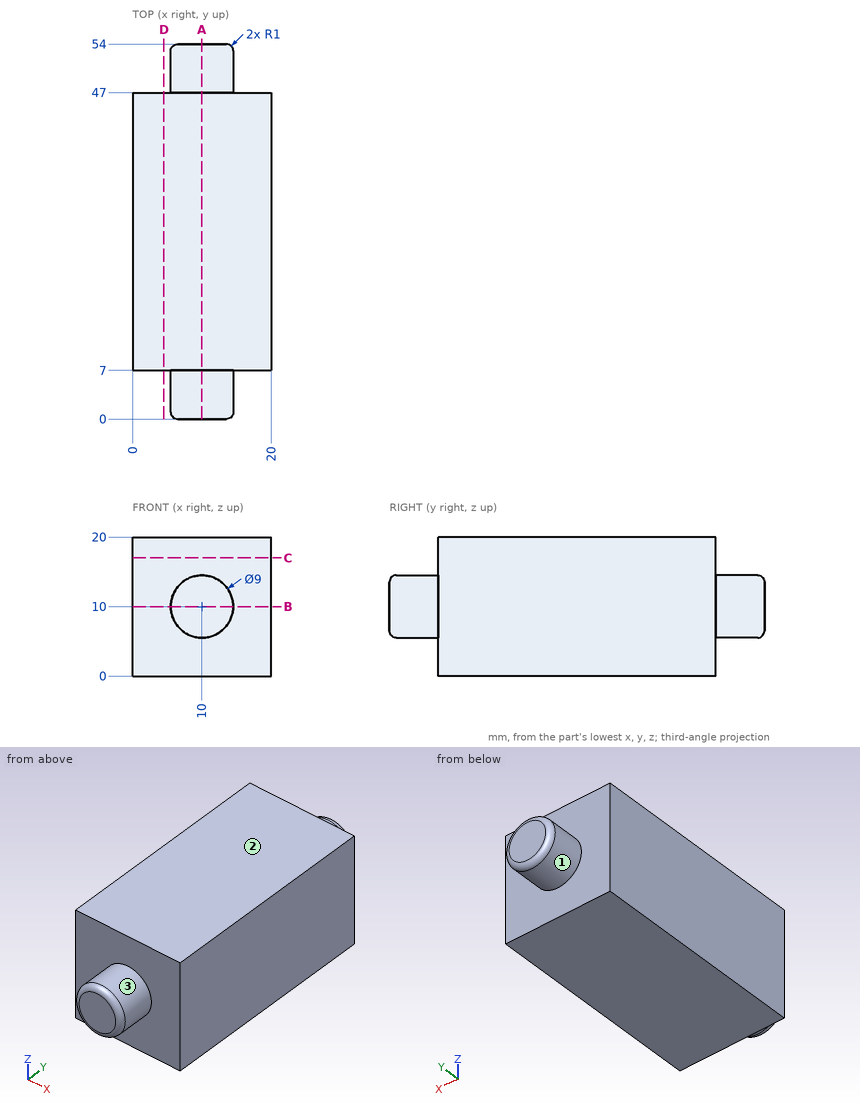
Source: three-view drawing plus pictorial views. Frame: mm from the lowest corner of the part. A direction names the side the tool comes from. Coordinates: 2 decimals unless noted, no trailing zeros. Order: outer loops, then holes, each group sorted by start corner. A loop starts at its lowest first (then second) coordinate and runs counter-clockwise, first axis right, second up. Notation, with made-up numbers: M 45.5,24.5 L 74.5,24.5 A32 cw 74.5,53.5 Z; hole C 47.5,49.5 d8. An arc over 180 degrees is marked long. Write each question's results on one line, items separated by ' | '. Start each with the question number.
1. Section D-D, the plane x = 4.5. Return the cut outline in (y, z).
2. Material intervals for L1, parallel to Y at x = 9.5, z = 19; L2, parallel to X at y = 49, z = 7, sorted ascending.
3. Reachability of the marked faces 1, 2 and 3 from +Z, -Z, +X, -X, +Y, -Y: full face, straight path, thin tool, end or side. Return the list, or none.
4. Section B-B, the plane z = 10. Return the cut outline in (x, y).
5. Pin query (flat end, axial travel): pin 1 (3 mm diameter, centred on x = 10, z = 16.5, fed in from -Y). Return the tip coordinate at first contact, or that it passes through.
6. Section C-C, the plane z = 17. Return the cut outline in (x, y).
7. Section A-A, the plane x = 10. Return the cut outline in (y, z), then the cut area to 3 significant figures.
Solution:
1) outline: M 7,0 L 47,0 L 47,20 L 7,20 Z
2) L1: 7 to 47 | L2: 6.65 to 13.35
3) face 1: +Y | face 2: +Z, +X, -X, +Y, -Y | face 3: -Y
4) outline: M 0,7 L 5.5,7 L 5.5,1 A1 ccw 6.5,0 L 13.5,0 A1 ccw 14.5,1 L 14.5,7 L 20,7 L 20,47 L 14.5,47 L 14.5,53 A1 ccw 13.5,54 L 6.5,54 A1 ccw 5.5,53 L 5.5,47 L 0,47 Z
5) pin 1: y = 7
6) outline: M 0,7 L 20,7 L 20,47 L 0,47 Z
7) outline: M 0,6.5 A1 ccw 1,5.5 L 7,5.5 L 7,0 L 47,0 L 47,5.5 L 53,5.5 A1 ccw 54,6.5 L 54,13.5 A1 ccw 53,14.5 L 47,14.5 L 47,20 L 7,20 L 7,14.5 L 1,14.5 A1 ccw 0,13.5 Z | area: 925 mm²
